Source: CAD feature listing. Evaluate the final solid. Frame: model axes, mm. Face numbers are marked on the shaded views. A direction names the side the tool comes from. Round coordinates to 2 decimals unless told otherwise and drop trailing zeros. Order: outer loops, then holes, each group sorted by start corner. A loop starts at its lowest first (then second) coordinate and runs counter-clockwise, first axis right, second up. Notation, with made-up numbers: (79.25, -10) - (113.25, -10) arc R29 ccw to (113.25, 21) - close; hole circle Ø9 at (74, -15). An arc over 180 degrees is marked (long way). Put each result on its own line as item: value. Start each with the question number.
1) Contact query for flat-ended pins moving along their axis: P1, Ø2, axis at x = -16, z = -4, coming from the -Y side; P2, Ø5, axis at y = 3.5, z = 2.5, coming from the -X side; P3, Ø4, axis at y = 4.5, z = 12, coming from the +X side; P4, Ø1.5, axis at x = 2, y = 7, coming from the -Z side. Output: stop coordinate, or through.
2) Section D-D on y = 3.5. Output: boundary loops of the cut face in (x, z).
3) Mould query, pull axis Z, two halves, no side actions, for the marked faces 1, 2 and 3. Classes: +Z half, -Z half, draft (parallel to the pull), parting line (faces both ways), or undercut.
4) Access query for the marked faces 4, 5 and 6. Directions: +Z, -Z, +X, -X, +Y, -Y. A direction counts if a zero-diameter tool reaches every point of the face in a straight line with its end or side. Return the directions, or none.
5) Section A-A on z = -18.75. Output: boundary loops of the cut face in (x, y).
6) Section C-C on x = 0. Output: boundary loops of the cut face in (y, z), then the cut area to 3 significant figures.
7) Line query: probe 1 along X at (y, z) = (2.05, 0); probe 2 along Z at (x, y) = (-10, 1.5); probe 3 along Y at (x, z) = (3, 16). Output: solid intervals per line, ascending. Write a range as [from, to].
8) Section B-B on x = -18.75. Output: boundary loops of the cut face in (y, z).
```python
from build123d import *

# Parameters (mm, degrees)
SKETCH_1_R          = 21.25
EXTRUDE_1_DEPTH     = 4
SKETCH_2_R          = 16.1
EXTRUDE_2_DEPTH     = 6
SKETCH_3_R          = 14
CUT_EXTRUDE_3_DEPTH = 8
SKETCH_4_R          = 6
CUT_EXTRUDE_4_DEPTH = 32.672148648
SKETCH_5_R          = 1.5
CUT_EXTRUDE_5_DEPTH = 10


with BuildPart() as part:
    # Эскиз1 → Вытянуть1 (new body)
    with BuildSketch(Plane(origin=(0, 0, 0), x_dir=(1, 0, 0), z_dir=(0, 1, 0))):
        with Locations(Location((0, 0, 0), (0, 0, 270))):
            Circle(SKETCH_1_R)
    extrude(amount=EXTRUDE_1_DEPTH)

    # Эскиз2 → Вытянуть2 (add)
    with BuildSketch(Plane(origin=(0, 4, 0), x_dir=(-1, 0, 0), z_dir=(0, 1, 0))):
        with Locations(Location((0, 0, 0), (0, 0, 90))):
            Circle(SKETCH_2_R)
    extrude(amount=EXTRUDE_2_DEPTH)

    # Эскиз3 → Вытянуть3 (cut)
    with BuildSketch(Plane.XZ):
        with Locations(Location((0, 0, 0), (0, 0, 270))):
            Circle(SKETCH_3_R)
    extrude(amount=-CUT_EXTRUDE_3_DEPTH, mode=Mode.SUBTRACT)

    # Эскиз4 → Вытянуть4 (cut, through all)
    with BuildSketch(Plane(origin=(0, 10, 0), x_dir=(1, 0, 0), z_dir=(0, 1, 0))):
        with Locations(Location((0, 0, 0), (0, 0, 270))):
            Circle(SKETCH_4_R)
    extrude(amount=-CUT_EXTRUDE_4_DEPTH, mode=Mode.SUBTRACT)

    # Эскиз5 → Вытянуть5 (cut)
    with BuildSketch(Plane(origin=(0, 4, 0), x_dir=(1, 0, 0), z_dir=(0, 1, 0))):
        with Locations(Location((0, 18.75, 0), (0, 0, 270))):
            Circle(SKETCH_5_R)
        with Locations(Location((18.75, 0, 0), (0, 0, 270))):
            Circle(SKETCH_5_R)
        with Locations(Location((0, -18.75, 0), (0, 0, 270))):
            Circle(SKETCH_5_R)
        with Locations(Location((-18.75, 0, 0), (0, 0, 270))):
            Circle(SKETCH_5_R)
    extrude(amount=-CUT_EXTRUDE_5_DEPTH, mode=Mode.SUBTRACT)


solid = part.part
```
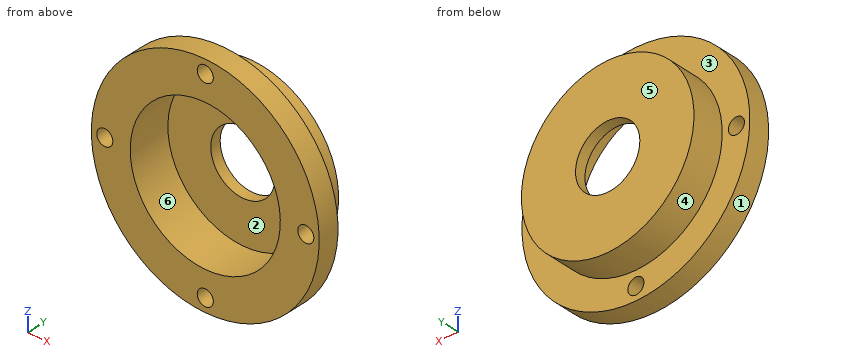
Answer sheet:
1. P1: y = 0
1. P2: x = -21.25
1. P3: x = 18.72
1. P4: z = -16.05
2. outline: circle Ø42.5 at (0, 0); hole circle Ø3 at (-18.75, 0); hole circle Ø28 at (0, 0); hole circle Ø3 at (0, -18.75); hole circle Ø3 at (0, 18.75); hole circle Ø3 at (18.75, 0)
3. face 1: parting line
3. face 2: undercut
3. face 3: draft
4. face 4: +Y
4. face 5: +Z, -Z, +X, -X, +Y
4. face 6: -Y
5. outline: (-10, 0) - (-1.5, 0) - (-1.5, 4) - (-10, 4) - close; (1.5, 0) - (10, 0) - (10, 4) - (1.5, 4) - close
6. outline: (0, -21.25) - (4, -21.25) - (4, -20.25) - (0, -20.25) - close; (0, -17.25) - (4, -17.25) - (4, -16.1) - (10, -16.1) - (10, -6) - (8, -6) - (8, -14) - (0, -14) - close; (0, 14) - (8, 14) - (8, 6) - (10, 6) - (10, 16.1) - (4, 16.1) - (4, 17.25) - (0, 17.25) - close; (0, 20.25) - (4, 20.25) - (4, 21.25) - (0, 21.25) - close
6. area: 91.2 mm^2
7. probe 1: [-21.25, -20.25], [-17.25, -14], [14, 17.25], [20.25, 21.25]
7. probe 2: [-18.75, -9.8], [9.8, 18.75]
7. probe 3: [0, 4]
8. outline: (0, -10) - (4, -10) - (4, -1.5) - (0, -1.5) - close; (0, 1.5) - (4, 1.5) - (4, 10) - (0, 10) - close
